Input: dimensioned drawing with shaded views. Units: mm. Origin: part minimum x, y, z. A direction names the side the tool comes from. Give positions to 0.01 mm unless a question says otherwise; leave off trailing zeros. Order: outer loops, then holes, each group sorted by start corner. A loop starts at its lowest first (then second) coordinate and runs counter-clockwise, first axis right, second up.
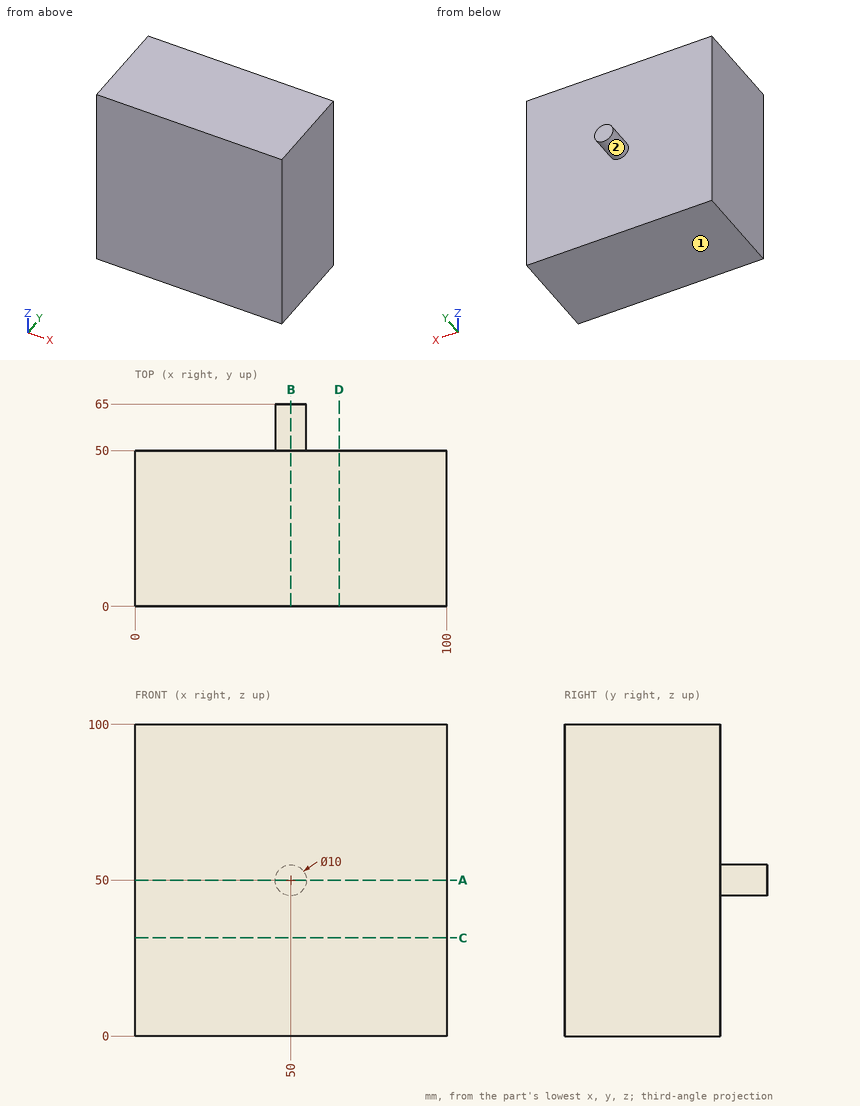
1) Section query A-A, the plane z = 50. Return the cut outline in (x, y).
Report:
outline: (0, 0) - (100, 0) - (100, 50) - (55, 50) - (55, 65) - (45, 65) - (45, 50) - (0, 50) - close
2) Pin query (flat end, axial travel): pin 1 (3 mm diameter, centred on x = 48.5, z = 18, fed in from +Y). Return the tip coordinate at first contact, or that it passes through.
Report:
pin 1: stops at y = 50
3) Material intervals for L1, parallel to Y at x = 40.5, z = 21; L2, parallel to Z at x = 50.5, y = 55.5, sorted ascending.
Report:
L1: y = 0 to 50
L2: z = 45.03 to 54.97
4) Reachability of the marked faces 1 and 2 from +Z, -Z, +X, -X, +Y, -Y: full face, straight path, thin tool, end or side. Return the list, or none.
Report:
face 1: -Z, +X, -X, +Y, -Y
face 2: +Y
5) Section query D-D, the plane x = 65.5. Return the cut outline in (y, z).
Report:
outline: (0, 0) - (50, 0) - (50, 100) - (0, 100) - close
6) Section query B-B, the plane x = 50. Return the cut outline in (y, z), and give its area (3 significant figures).
Report:
outline: (0, 0) - (50, 0) - (50, 45) - (65, 45) - (65, 55) - (50, 55) - (50, 100) - (0, 100) - close
area: 5,150 mm2
7) Section query C-C, the plane z = 31.5. Return the cut outline in (x, y).
Report:
outline: (0, 0) - (100, 0) - (100, 50) - (0, 50) - close
